Verification items for the finished model (mm, model axes). Face numbers are marked on the shaded views. Give positions to 0.01 mm unless a question says otherwise; leave off trailing zeros. Order: outer loops, then holes, each group sorted by start corner. A loop starts at its lowest first (then second) coordinate and runs counter-clockwise, first axis right, second up. Notation, with made-up numbers: M 72.25,-29.75 L 90.25,-29.75 A25 ccw 90.25,-8.75 Z; hole C 84.5,-39 d7. An arc over 180 degrees is marked long. Answer as a JSON object with one key per item and string values.
```python
from build123d import *

# Parameters (mm, degrees)
SKETCH1_W            = 178
SKETCH1_H            = 150
BOSS_EXTRUDE1_DEPTH  = 6
SKETCH2_W            = 6
SKETCH2_H            = 25
CUT_EXTRUDE1_DEPTH   = 6
LPATTERN1_COUNT      = 3
LPATTERN1_PITCH      = 50
LPATTERN1_COUNT_DIR2 = 2
LPATTERN1_PITCH_DIR2 = 172


with BuildPart() as part:
    # Sketch1 → Boss-Extrude1 (new body)
    with BuildSketch(Plane.XY):
        with Locations((-89, 75)):
            Rectangle(SKETCH1_W, SKETCH1_H)
    extrude(amount=BOSS_EXTRUDE1_DEPTH)

    # Sketch2 → Cut-Extrude1 (cut)
    with BuildSketch(Plane.XY.offset(6)):
        with Locations((-175, 112.5)):
            Rectangle(SKETCH2_W, SKETCH2_H)
    cut_extrude1 = extrude(amount=-CUT_EXTRUDE1_DEPTH, mode=Mode.SUBTRACT)

    # LPattern1: Cut-Extrude1 3 × 2
    with Locations(*[(j * LPATTERN1_PITCH_DIR2, -i * LPATTERN1_PITCH, 0) for i in range(LPATTERN1_COUNT) for j in range(LPATTERN1_COUNT_DIR2) if (i, j) != (0, 0)]):
        add(cut_extrude1, mode=Mode.SUBTRACT)


solid = part.part
```
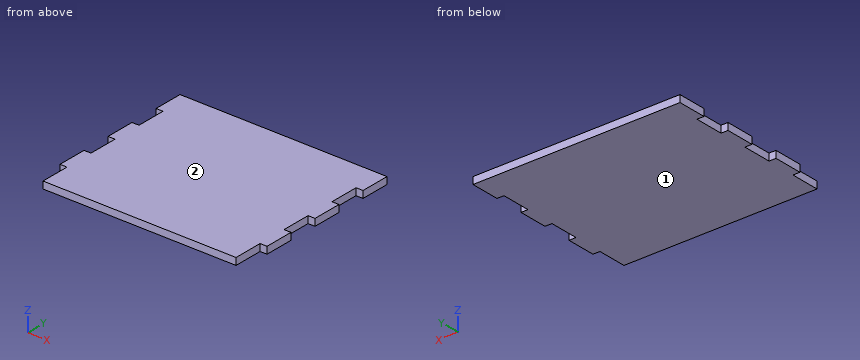
Q1. Section check A-A on z = 2.1. Record the cut outline in (x, y).
Resolved:
{"outline": "M -178,25 L -172,25 L -172,0 L -6,0 L -6,25 L 0,25 L 0,50 L -6,50 L -6,75 L 0,75 L 0,100 L -6,100 L -6,125 L 0,125 L 0,150 L -178,150 L -178,125 L -172,125 L -172,100 L -178,100 L -178,75 L -172,75 L -172,50 L -178,50 Z"}
Q2. Material ranges on L1, parallel to X at y = 110, z = 2.8, recorded low to high.
Resolved:
{"L1": "x = -172 to -6"}
Q3. Gauge pin test, flat ends, axial feed: pin 1 Ø1.5 at (y, z) = (115.5, 2.5) entering from +X; pin 2 Ø1.8 at (x, z) = (-4, 1.5) entering from -Y; pin 3 Ø1.5 at (y, z) = (118.5, 0.5) entering from -X. Record the tip position at first contact, or that the pin passes through.
Resolved:
{"pin 1": "stops at x = -6", "pin 2": "stops at y = 25", "pin 3": "stops at x = -172"}
Q4. Release check for a two-part mould opening along Z. For the marked faces 1 and 2 record: +Z half, -Z half, draft (parallel to the pull), parting line (faces both ways), or undercut.
Resolved:
{"face 1": "-Z half", "face 2": "+Z half"}
Q5. Section check B-B on y = 69. Record the cut outline in (x, z).
Resolved:
{"outline": "M -172,0 L -6,0 L -6,6 L -172,6 Z"}
